Could you check a few things on this model? Use its own coordinates, in mm. A direction names the side the tool comes from. Give positions to 0.01 mm unless a question says otherwise; leave off trailing zeros. Loops run counter-clockwise (first coordinate to the right, second up) from the corner with the lowest first, then second, coordinate; pieces in that order, holes last.
1. For faces 5 (the flat face through (16, 0, -2)), 6 (the flat face through (-17, 0, 8)), 7 (the flat face through (-16, 0, -2)), which set-ups out of +Z, -Z, +X, -X, +Y, -Y let a thin tool reach every point of the face, with its end or its side?
2. Imagine slicing it at A-A (y = 9). List the corners of the cut face in (x, z) for me, plus the area to 3 significant figures.
3. Thinking about a two-plate mould opening in X: for faces 1 (the flat face through (16.49, -0.21, 4.28)), 2 (the cylindrical face through (-13.27, 8.03, 2.13)), 3 (the cylindrical face through (10.4, -8.93, 2.13)), 4 (the flat face through (-4, -15, 5)), which applies, +X half, -X half, draft (parallel to the pull), parting line (faces both ways), or undercut?
4. Imagine slicing it at D-D (y = 1.75). List the corners of the cut face in (x, z) for me.
5. Imagine slicing it at C-C (x = -12). List the corners of the cut face in (y, z) for me, plus the area to 3 significant figures.
6. I need wall thicknesses on line 1 along Y through (x, z) = (12, 1.5); line 2 along Z through (x, y) = (0, -4.75); line 3 along Z through (x, y) = (-9.5, -5.75). Which ranges of each line are inside material? Lowest first, please.
7. For P1, Ø4, axis at x = -11.5, y = 0, coming from the -Z side; P2, Ø1.9, axis at x = 12, y = 9, coming from the +Z side; P3, Ø12, axis at y = -3, z = -8.5, coming from the -X side; P4, Ø1.5, axis at x = -1.5, y = 9, coming from the -Z side, each with a flat end and sliding along its axis, tell me the tip position at first contact or that it passes through.
8. Imagine slicing it at B-B (z = 0). List the corners of the cut face in (x, y) for me.
```python
from build123d import *

# Parameters (mm, degrees)
F0_R     = 5
F1_DEPTH = 15
F2_R     = 1.6
F3_DEPTH = 25


with BuildPart() as f1:
    # F0 (on Front) → F1 (new body, symmetric)
    with BuildSketch(Plane.XZ):
        with BuildLine():
            Line((-16, -7), (-8.485281, -7))
            ThreePointArc((-8.485281, -7), (0, -11), (8.485281, -7))
            Line((8.485281, -7), (16, -7))
            Line((16, -7), (16, 3.584423))
            Line((16, 3.584423), (17, 5))
            Line((17, 5), (17, 11))
            Line((17, 11), (0, 11))
            Line((0, 11), (-17, 11))
            Line((-17, 11), (-17, 5))
            Line((-17, 5), (-16, 3.584423))
            Line((-16, 3.584423), (-16, -7))
        make_face()
        Circle(F0_R, mode=Mode.SUBTRACT)
    extrude(amount=F1_DEPTH, both=True)

    # F2 (on face) → F3 (cut)
    with BuildSketch(Plane.XY.offset(11)):
        with Locations((-12, -9)):
            Circle(F2_R)
        with Locations((12, -9)):
            Circle(F2_R)
        with Locations((12, 9)):
            Circle(F2_R)
        with Locations((-12, 9)):
            Circle(F2_R)
    extrude(amount=-F3_DEPTH, mode=Mode.SUBTRACT)


solid = f1.part
```
Derived:
1. face 5: -Z, +X, +Y, -Y
1. face 6: +Z, -Z, -X, +Y, -Y
1. face 7: -Z, -X, +Y, -Y
2. outline: (-17, 5) - (-16, 3.58) - (-16, -7) - (-13.6, -7) - (-13.6, 11) - (-17, 11) - close; (-10.4, -7) - (-8.49, -7) arc R11 ccw to (8.49, -7) - (10.4, -7) - (10.4, 11) - (-10.4, 11) - close; (13.6, -7) - (16, -7) - (16, 3.58) - (17, 5) - (17, 11) - (13.6, 11) - close; hole circle Ø10 at (0, 0)
2. area: 443 mm2
3. face 1: +X half
3. face 2: undercut
3. face 3: undercut
3. face 4: draft
4. outline: (-17, 5) - (-16, 3.58) - (-16, -7) - (-8.49, -7) arc R11 ccw to (8.49, -7) - (16, -7) - (16, 3.58) - (17, 5) - (17, 11) - (-17, 11) - close; hole circle Ø10 at (0, 0)
5. outline: (-15, -7) - (-10.6, -7) - (-10.6, 11) - (-15, 11) - close; (-7.4, -7) - (7.4, -7) - (7.4, 11) - (-7.4, 11) - close; (10.6, -7) - (15, -7) - (15, 11) - (10.6, 11) - close
5. area: 425 mm2
6. line 1: y = -15 to -10.6, -7.4 to 7.4, 10.6 to 15
6. line 2: z = -11 to -5, 5 to 11
6. line 3: z = -7 to 11
7. P1: stops at z = -7
7. P2: passes through
7. P3: stops at x = -16
7. P4: stops at z = -10.97
8. outline: (-16, -15) - (-5, -15) - (-5, 15) - (-16, 15) - close; (5, -15) - (16, -15) - (16, 15) - (5, 15) - close; hole circle Ø3.2 at (-12, -9); hole circle Ø3.2 at (-12, 9); hole circle Ø3.2 at (12, -9); hole circle Ø3.2 at (12, 9)
